```python
from build123d import *

# Parameters (mm, degrees)
SKETCH1_W           = 42
SKETCH1_H           = 42
BOSS_EXTRUDE1_DEPTH = 40
CHAMFER1_SIZE       = 5
SKETCH2_R           = 11
BOSS_EXTRUDE3_DEPTH = 2
SKETCH5_R           = 2.5
BOSS_EXTRUDE4_DEPTH = 4
SKETCH6_R           = 8
BOSS_EXTRUDE5_DEPTH = 7
SKETCH7_R           = 6
BOSS_EXTRUDE6_DEPTH = 7
SKETCH8_R           = 8
BOSS_EXTRUDE7_DEPTH = 1.5
SKETCH9_R           = 1.5
CUT_EXTRUDE1_DEPTH  = 4.5
SKETCH10_W          = 4
SKETCH10_H          = 4
BOSS_EXTRUDE8_DEPTH = 10


with BuildPart() as part:
    # Sketch1 → Boss-Extrude1 (new body)
    with BuildSketch(Plane(origin=(0, 0, 0), x_dir=(1, 0, 0), z_dir=(0, 1, 0))):
        Rectangle(SKETCH1_W, SKETCH1_H)
    extrude(amount=BOSS_EXTRUDE1_DEPTH)

    # Chamfer1
    chamfer1_edges = [part.edges().sort_by_distance(p)[0] for p in [
        (21, 20, 21),
        (-21, 20, 21),
        (-21, 20, -21),
        (21, 20, -21),
    ]]
    chamfer(chamfer1_edges, length=CHAMFER1_SIZE)

    # Sketch2 → Boss-Extrude3 (add)
    with BuildSketch(Plane(origin=(0, 40, 0), x_dir=(1, 0, 0), z_dir=(0, 1, 0))):
        with Locations(Location((0, 0, 0), (0, 0, 270))):
            Circle(SKETCH2_R)
    extrude(amount=BOSS_EXTRUDE3_DEPTH)

    # Sketch5 → Boss-Extrude4 (add)
    with BuildSketch(Plane(origin=(0, 42, 0), x_dir=(1, 0, 0), z_dir=(0, 1, 0))):
        with Locations(Location((0, 0, 0), (0, 0, 270))):
            Circle(SKETCH5_R)
    extrude(amount=BOSS_EXTRUDE4_DEPTH)

    # Sketch6 → Boss-Extrude5 (add)
    with BuildSketch(Plane(origin=(0, 46, 0), x_dir=(1, 0, 0), z_dir=(0, 1, 0))):
        with Locations(Location((0, 0, 0), (0, 0, 270))):
            Circle(SKETCH6_R)
    extrude(amount=BOSS_EXTRUDE5_DEPTH)

    # Sketch7 → Boss-Extrude6 (add)
    with BuildSketch(Plane(origin=(0, 53, 0), x_dir=(1, 0, 0), z_dir=(0, 1, 0))):
        with Locations(Location((0, 0, 0), (0, 0, 270))):
            Circle(SKETCH7_R)
    extrude(amount=BOSS_EXTRUDE6_DEPTH)

    # Sketch8 → Boss-Extrude7 (add)
    with BuildSketch(Plane(origin=(0, 60, 0), x_dir=(1, 0, 0), z_dir=(0, 1, 0))):
        with Locations(Location((0, 0, 0), (0, 0, 270))):
            Circle(SKETCH8_R)
    extrude(amount=BOSS_EXTRUDE7_DEPTH)

    # Sketch9 → Cut-Extrude1 (cut)
    with BuildSketch(Plane(origin=(0, 40, 0), x_dir=(1, 0, 0), z_dir=(0, 1, 0))):
        with Locations(Location((-15.5, 15.5, 0), (0, 0, 270))):
            Circle(SKETCH9_R)
        with Locations(Location((15.5, 15.5, 0), (0, 0, 270))):
            Circle(SKETCH9_R)
        with Locations(Location((15.5, -15.5, 0), (0, 0, 270))):
            Circle(SKETCH9_R)
        with Locations(Location((-15.5, -15.5, 0), (0, 0, 270))):
            Circle(SKETCH9_R)
    extrude(amount=-CUT_EXTRUDE1_DEPTH, mode=Mode.SUBTRACT)

    # Sketch10 → Boss-Extrude8 (add)
    with BuildSketch(Plane.XY.offset(21)):
        with Locations((0, 6.6)):
            Rectangle(SKETCH10_W, SKETCH10_H)
    extrude(amount=BOSS_EXTRUDE8_DEPTH)


solid = part.part
```
Can you work these out from the model? Positions are in its coordinate system, mm. A direction names the side the tool comes from. Coordinates: 2 decimals unless noted, no trailing zeros. Loops run counter-clockwise (first coordinate to the right, second up) from the corner with the lowest first, then second, coordinate; pieces in that order, holes last. Notation, with made-up numbers: M 55.25,77.25 L 96.25,77.25 A18 ccw 96.25,107.25 Z; hole C 70,83.5 d9. An arc over 180 degrees is marked long. Put each result on its own line as item: value. Start each with the question number.
(1) Will these pins go through, and if not, where does the flat tip stop? pin 1 Ø1.2 at (y, z) = (5.5, 27) entering from +X; pin 2 Ø4.5 at (x, z) = (1, 27) entering from -Y; pin 3 Ø0.9 at (x, z) = (-16, 15) entering from +Y.
(2) Imagine slicing it at A-A on z = 0. List the corners of the cut face in (x, y) for me, and give its area (3 significant figures).
(3) Imagine slicing it at C-C on y = 14.5. List the corners of the cut face in (x, z) for me.
(4) Which directions (+Z, -Z, +X, -X, +Y, -Y) give clear straight access to the entire face, cutting with the end or side of a thin tool? Please do faces 4 (the face through (0, 4.6, 26)), 5 (the face through (-2, 7, 26)), 6 (the face through (6, 60, -2)), 7 (the face through (-15.43, 37.78, -17)), 8 (the face through (0, 8.6, 26)).
(5) I need wall thicknesses on probe 1 along X at (y, z) = (38.35, -15.5); probe 2 along Y at (x, z) = (-1, -6); probe 3 along X at (y, z) = (38, -15). Which ranges of each line are inside material? Lowest first, please.
(6) Imagine slicing it at B-B on x = 0. List the corners of the cut face in (y, z) for me.
(7) We'd pull the mould along Y, two halves only. Please class faces 1 (the face through (19, 20, 18)), 2 (the face through (16, 35.5, -16)), 3 (the face through (-2.44, 43.97, -0.54)): +Y half, -Y half, draft (parallel to the pull), parting line (faces both ways), or undercut.
(8) Imagine slicing it at D-D on x = 7. List the corners of the cut face in (y, z) for me.
Worked answers:
1. pin 1: stops at x = 2
1. pin 2: stops at y = 4.6
1. pin 3: stops at y = 35.5
2. outline: M -21,0 L 21,0 L 21,40 L 11,40 L 11,42 L 2.5,42 L 2.5,46 L 8,46 L 8,53 L 6,53 L 6,60 L 8,60 L 8,61.5 L -8,61.5 L -8,60 L -6,60 L -6,53 L -8,53 L -8,46 L -2.5,46 L -2.5,42 L -11,42 L -11,40 L -21,40 Z
2. area: 1,960 mm2
3. outline: M -21,-16 L -16,-21 L 16,-21 L 21,-16 L 21,16 L 16,21 L -16,21 L -21,16 Z
4. face 4: +Z, +X, -X, -Y
4. face 5: +Z, -X, +Y, -Y
4. face 6: none
4. face 7: +Y
4. face 8: +Z, +X, -X, +Y
5. probe 1: x = -21 to -17, -14 to 14, 17 to 21
5. probe 2: y = 0 to 42, 46 to 53, 60 to 61.5
5. probe 3: x = -21 to -16.91, -14.09 to 14.09, 16.91 to 21
6. outline: M 0,-21 L 40,-21 L 40,-11 L 42,-11 L 42,-2.5 L 46,-2.5 L 46,-8 L 53,-8 L 53,-6 L 60,-6 L 60,-8 L 61.5,-8 L 61.5,8 L 60,8 L 60,6 L 53,6 L 53,8 L 46,8 L 46,2.5 L 42,2.5 L 42,11 L 40,11 L 40,21 L 8.6,21 L 8.6,31 L 4.6,31 L 4.6,21 L 0,21 Z
7. face 1: draft
7. face 2: +Y half
7. face 3: undercut
8. outline: M 0,-21 L 40,-21 L 40,-8.49 L 42,-8.49 L 42,8.49 L 40,8.49 L 40,21 L 0,21 Z; M 46,-3.87 L 53,-3.87 L 53,3.87 L 46,3.87 Z; M 60,-3.87 L 61.5,-3.87 L 61.5,3.87 L 60,3.87 Z
